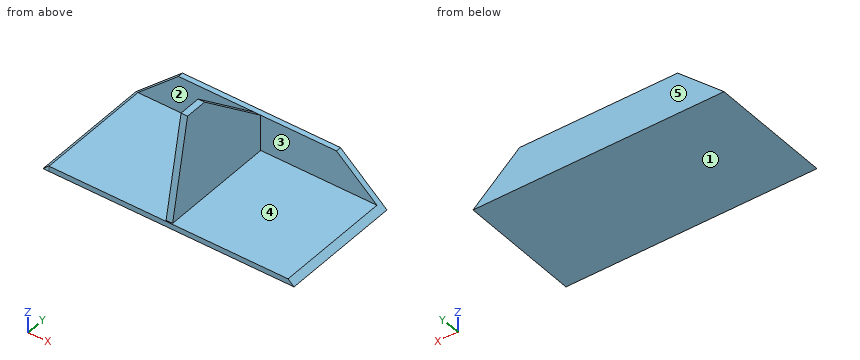
```python
from build123d import *

# Parameters (mm, degrees)
SKETCH_1_W          = 540
SKETCH_1_H          = 265
SKETCH_1_R          = 13
EXTRUDE_635_DEPTH   = 11.5
SKETCH_2_W          = 540
SKETCH_2_H          = 11.5
EXTRUDE_1_DEPTH     = 77.5
CUT_EXTRUDE_1_DEPTH = 609.067430471
SKETCH_4_R          = 13
CUT_EXTRUDE_2_DEPTH = 609.067430471
SKETCH_5_W          = 14
SKETCH_5_H          = 253.5
EXTRUDE_2_DEPTH     = 208.5
SKETCH_6_R          = 13
CUT_EXTRUDE_3_DEPTH = 442.988687638
EXTRUDE_3_DEPTH     = 14
SKETCH_8_W          = 514.15730337
SKETCH_8_H          = 253.5
EXTRUDE_4_DEPTH     = 11.5
EXTRUDE_5_DEPTH     = 11.5


with BuildPart() as part:
    # Sketch 1 → Extrude 635 (new body)
    with BuildSketch(Plane.XY):
        with Locations((270, 132.5)):
            Rectangle(SKETCH_1_W, SKETCH_1_H)
        with Locations((97.46594539, 108.46594539)):
            Circle(SKETCH_1_R, mode=Mode.SUBTRACT)
        with Locations((40.897402896, 51.897402896)):
            Circle(SKETCH_1_R, mode=Mode.SUBTRACT)
        with Locations(Location((499.102597104, 51.897402896, 0), (0, 0, 180))):
            Circle(SKETCH_1_R, mode=Mode.SUBTRACT)
        with Locations(Location((402.170987639, 92.261534081, 0), (0, 0, 180))):
            Circle(SKETCH_1_R, mode=Mode.SUBTRACT)
        with Locations((230, 121)):
            Circle(SKETCH_1_R, mode=Mode.SUBTRACT)
        with Locations((230, 41)):
            Circle(SKETCH_1_R, mode=Mode.SUBTRACT)
        with Locations(Location((310, 41, 0), (0, 0, 180))):
            Circle(SKETCH_1_R, mode=Mode.SUBTRACT)
        with Locations(Location((310, 121, 0), (0, 0, 180))):
            Circle(SKETCH_1_R, mode=Mode.SUBTRACT)
        with Locations((137.829012361, 92.261534081)):
            Circle(SKETCH_1_R, mode=Mode.SUBTRACT)
        with Locations(Location((442.53405461, 108.46594539, 0), (0, 0, 180))):
            Circle(SKETCH_1_R, mode=Mode.SUBTRACT)
    extrude(amount=EXTRUDE_635_DEPTH)

    # Sketch 2 → Extrude 1 (add)
    with BuildSketch(Plane.XY.offset(11.5)):
        with Locations((270, 259.25)):
            Rectangle(SKETCH_2_W, SKETCH_2_H)
    extrude(amount=EXTRUDE_1_DEPTH)

    # Sketch 3 → Cut-Extrude 1 (cut, through all)
    with BuildSketch(Plane(origin=(0, 265, 0), x_dir=(-1, 0, 0), z_dir=(0, 1, 0))):
        Polygon((0, 0), (-100, 89), (0, 89), align=None)
        Polygon((-540, 0), (-440, 89), (-540, 89), align=None)
    extrude(amount=-CUT_EXTRUDE_1_DEPTH, mode=Mode.SUBTRACT)

    # Sketch 4 → Cut-Extrude 2 (cut, through all)
    with BuildSketch(Plane(origin=(0, 265, 0), x_dir=(-1, 0, 0), z_dir=(0, 1, 0))):
        with Locations(Location((-210, 50, 0), (0, 0, 90))):
            Circle(SKETCH_4_R)
        with Locations(Location((-130, 50, 0), (0, 0, 90))):
            Circle(SKETCH_4_R)
        with Locations(Location((-410, 50, 0), (0, 0, 90))):
            Circle(SKETCH_4_R)
        with Locations(Location((-330, 50, 0), (0, 0, 90))):
            Circle(SKETCH_4_R)
    extrude(amount=-CUT_EXTRUDE_2_DEPTH, mode=Mode.SUBTRACT)

    # Sketch 5 → Extrude 2 (add)
    with BuildSketch(Plane.XY.offset(11.5)):
        with Locations((270, 126.75)):
            Rectangle(SKETCH_5_W, SKETCH_5_H)
    extrude(amount=EXTRUDE_2_DEPTH)

    # Sketch 6 → Cut-Extrude 3 (cut, through all)
    with BuildSketch(Plane(origin=(277, 0, 0), x_dir=(0, 0, -1), z_dir=(1, 0, 0))):
        with Locations((-115.676148082, 138.142814541)):
            Circle(SKETCH_6_R)
        with Locations((-175.462621788, 84.986652509)):
            Circle(SKETCH_6_R)
        with Locations((-68.377294113, 126.911974174)):
            Circle(SKETCH_6_R)
        Polygon((-89, 253.5), (-220, 93.5), (-220, 253.5), align=None)
        Polygon((-220, 45), (0, 0), (-220, 0), align=None)
    extrude(amount=-CUT_EXTRUDE_3_DEPTH, mode=Mode.SUBTRACT)

    # Sketch 7 → Extrude 3 (add)
    with BuildSketch(Plane(origin=(277, 0, 0), x_dir=(0, 0, -1), z_dir=(1, 0, 0))):
        Polygon((-220, 93.5), (-220, 45), (-11.5, 2.352272727), (-11.5, 253.5), (-89, 253.5), align=None)
    extrude(amount=-EXTRUDE_3_DEPTH)

    # Sketch 8 → Extrude 4 (add)
    with BuildSketch(Plane.XY.offset(11.5)):
        with Locations((270, 126.75)):
            Rectangle(SKETCH_8_W, SKETCH_8_H)
    extrude(amount=-EXTRUDE_4_DEPTH)

    # Sketch 9 → Extrude 5 (add)
    with BuildSketch(Plane(origin=(0, 265, 0), x_dir=(1, 0, 0), z_dir=(0, 1, 0))):
        Polygon((0, 0), (100, -89), (440, -89), (540, 0), align=None)
    extrude(amount=-EXTRUDE_5_DEPTH)


solid = part.part
```
The listing builds one solid part. Answer for the finished solid, in the listing's coordinates (mm). Face numbers are marked on the shaded views. A direction names the side the tool comes from. Coordinates: 2 decimals unless noted, no trailing zeros. Write each loop counter-clockwise with the first axis right and the second up, starting at its lowest first coordinate (ties: lowest second). Pieces come first, ordered by that corner, then holes.
Q1. Section C-C, the plane y = 108.5 is taken. Write down the section's boundary in (x, z), then the cut area to 3 significant figures.
Returned:
outline: (0, 0) - (540, 0) - (527.08, 11.5) - (277, 11.5) - (277, 207.72) - (263, 207.72) - (263, 11.5) - (12.92, 11.5) - close
area: 8,810 mm2
Q2. Section D-D, the plane x = 215.5 is taken. Write down the section's boundary in (y, z).
Returned:
outline: (0, 0) - (265, 0) - (265, 89) - (253.5, 89) - (253.5, 11.5) - (0, 11.5) - close
Q3. Section A-A, the plane x = 480 is taken. Write down the section's boundary in (y, z), then the cut area to 3 significant figures.
Returned:
outline: (0, 0) - (265, 0) - (265, 53.4) - (253.5, 53.4) - (253.5, 11.5) - (0, 11.5) - close
area: 3,530 mm2
Q4. Which of the six approach directions +Z, -Z, +X, -X, +Y, -Y give full straight-line access (tool end or side, diameter ignored) to the marked faces 1, 2, 3, 4 and 5?
Returned:
face 1: -Z, +X, -X, +Y, -Y
face 2: +Z, -X, -Y
face 3: +Z, +X, -Y
face 4: +Z, -Y
face 5: +Z, -Z, +X, -X, +Y
Q5. Given P1, Ø8, axis at y = 76, z = 99, coming from the +X side; P2, Ø2, axis at y = 44.5, z = 152, coming from the -X side; P3, Ø0.7, axis at y = 1.5, z = 3, coming from the -X side, each flat-ended and moving along its own axis, determine where each tip first touches the part or whether it passes through.
Returned:
P1: stops at x = 277
P2: stops at x = 263
P3: stops at x = 2.98
Q6. Section B-B, the plane z = 50.5 is taken. Write down the section's boundary in (x, y).
Returned:
outline: (56.74, 253.5) - (263, 253.5) - (263, 10.33) - (277, 10.33) - (277, 253.5) - (483.26, 253.5) - (483.26, 265) - (56.74, 265) - close
Q7. Find the intervals of material crossed by line 1 along X through (y, z) = (76.5, 106.5); line 2 along Z through (x, y) = (278, 170); line 3 along Z through (x, y) = (267.5, 254), in increasing order.
Returned:
line 1: x = 263 to 277
line 2: z = 0 to 11.5
line 3: z = 0 to 89
